from build123d import *

# Parameters (mm, degrees)
SKETCH_1_R          = 1.2
EXTRUDE_1_DEPTH     = 3
EXTRUDE_2_DEPTH     = 200
FILLET_1_R          = 4
SKETCH_4_W          = 24.434656606
SKETCH_4_H          = 24.505426632
CUT_EXTRUDE_1_DEPTH = 4
FILLET_3_R          = 8
SKETCH_5_W          = 15
SKETCH_5_H          = 20
CUT_EXTRUDE_2_DEPTH = 10
FILLET_4_R          = 10
FILLET_5_R          = 10


with BuildPart() as part:
    # 草图1 → 凸台-拉伸1 (new body)
    with BuildSketch(Plane.XY):
        Polygon((-68.534318099, 4.283164377), (-80.94435421, -20.816457208), (-55.844732625, -33.22649332), (-43.434696514, -8.126871734), align=None)
        with Locations((-66.577549394, -0.711768645)):
            Circle(SKETCH_1_R, mode=Mode.SUBTRACT)
        with Locations((-75.441860902, -18.640069777)):
            Circle(SKETCH_1_R, mode=Mode.SUBTRACT)
        with Locations((-57.51355977, -27.504381286)):
            Circle(SKETCH_1_R, mode=Mode.SUBTRACT)
        with Locations((-48.649248262, -9.576080153)):
            Circle(SKETCH_1_R, mode=Mode.SUBTRACT)
    extrude(amount=EXTRUDE_1_DEPTH)

    # 草图2 → 凸台-拉伸2 (add)
    with BuildSketch(Plane.XY.offset(3)):
        Polygon((-86.606649797, -63.783530386), (-38.474241258, 35.126889936), (-35.77668434, 33.814187885), (-83.909092879, -65.096232437), align=None)
    extrude(amount=EXTRUDE_2_DEPTH)

    # 圆角1
    fillet_1_edges = [part.edges().sort_by_distance(p)[0] for p in [
        (-59.839316246, -15.633681193, 3),
        (-62.528614635, -14.304008154, 3),
    ]]
    fillet(fillet_1_edges, radius=FILLET_1_R)

    # 草图4 → 切除-拉伸1 (cut)
    with BuildSketch(Plane(origin=(-44.928588602, 21.863431321, 0), x_dir=(0, 0, 1), z_dir=(-0.8991856392880848, 0.43756735035658034, 0))):
        with Locations((15.217328303, -82.996763505)):
            Rectangle(SKETCH_4_W, SKETCH_4_H)
    extrude(amount=-CUT_EXTRUDE_1_DEPTH, mode=Mode.SUBTRACT)

    # 圆角3
    fillet_3_edges = [part.edges().sort_by_distance(p)[0] for p in [
        (-74.535096738, -42.4049537, 3),
        (-74.535096738, -42.4049537, 27.434656606),
    ]]
    fillet(fillet_3_edges, radius=FILLET_3_R)

    # 草图5 → 切除-拉伸2 (cut)
    with BuildSketch(Plane(origin=(-42.231031684, 20.55072927, 0), x_dir=(0, 0, -1), z_dir=(0.8991856392880848, -0.4375673503565804, 0))):
        with Locations((-60.064574797, -10.249476821)):
            Rectangle(SKETCH_5_W, SKETCH_5_H)
        with Locations((-29.955718497, -10.249476821)):
            Rectangle(SKETCH_5_W, SKETCH_5_H)
        with Locations((-90.173431098, -10.249476821)):
            Rectangle(SKETCH_5_W, SKETCH_5_H)
        with Locations((-120.282287399, -10.249476821)):
            Rectangle(SKETCH_5_W, SKETCH_5_H)
        with Locations((-150.391143699, -10.249476821)):
            Rectangle(SKETCH_5_W, SKETCH_5_H)
        with Locations((-180.5, -10.249476821)):
            Rectangle(SKETCH_5_W, SKETCH_5_H)
        with Locations((-60.064574797, -40.249476821)):
            Rectangle(SKETCH_5_W, SKETCH_5_H)
        with Locations((-90.173431098, -40.249476821)):
            Rectangle(SKETCH_5_W, SKETCH_5_H)
        with Locations((-120.282287399, -40.249476821)):
            Rectangle(SKETCH_5_W, SKETCH_5_H)
        with Locations((-150.391143699, -40.249476821)):
            Rectangle(SKETCH_5_W, SKETCH_5_H)
        with Locations((-180.5, -40.249476821)):
            Rectangle(SKETCH_5_W, SKETCH_5_H)
        with Locations((-60.064574797, -70.249476821)):
            Rectangle(SKETCH_5_W, SKETCH_5_H)
        with Locations((-90.173431098, -70.249476821)):
            Rectangle(SKETCH_5_W, SKETCH_5_H)
        with Locations((-120.282287399, -70.249476821)):
            Rectangle(SKETCH_5_W, SKETCH_5_H)
        with Locations((-150.391143699, -70.249476821)):
            Rectangle(SKETCH_5_W, SKETCH_5_H)
        with Locations((-180.5, -70.249476821)):
            Rectangle(SKETCH_5_W, SKETCH_5_H)
        with Locations((-29.955718497, -40.249476821)):
            Rectangle(SKETCH_5_W, SKETCH_5_H)
    extrude(amount=-CUT_EXTRUDE_2_DEPTH, mode=Mode.SUBTRACT)

    # 圆角4
    fillet_4_edges = [part.edges().sort_by_distance(p)[0] for p in [
        (-37.125462799, 34.470538911, 203),
    ]]
    fillet(fillet_4_edges, radius=FILLET_4_R)

    # 圆角5
    fillet_5_edges = [part.edges().sort_by_distance(p)[0] for p in [
        (-37.125462799, 34.470538911, 3),
    ]]
    fillet(fillet_5_edges, radius=FILLET_5_R)


solid = part.part
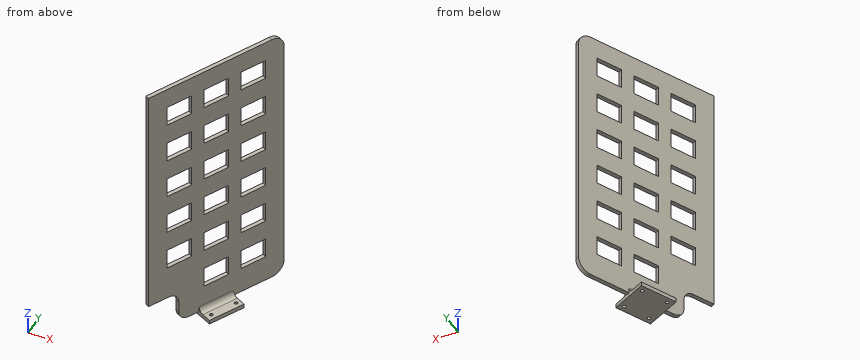
Source: CAD feature listing. Evaluate the final solid. Frame: model axes, mm. Give positions to 0.01 mm unless a question says otherwise; leave off trailing zeros. Write each loop counter-clockwise with the first axis right and the second up, starting at its lowest first coordinate (ties: lowest second). Pieces come first, ordered by that corner, then holes. Notation, with made-up numbers: M -17.75,-18 L -0.75,-18 A18 ccw -0.75,-6 Z; hole C 81.5,39 d4. An arc over 180 degrees is marked long. Return JSON: item names as keys, results as strings. Group by question number.
1) Cut plane B-B, the plane y = 15. Output: boundary loops of the cut face in (x, z), plus the area to 3 significant figures.
2) Pin query (flat end, axial travel): P1, Ø3, axis at x = -48.65, y = -9.58, coming from the +Z side; P2, Ø3.5, axis at x = -45.5, y = 11, coming from the -Z side; P3, Ø3.5, axis at x = -74.5, y = -42.5, coming from the -Z side. Return the tip coordinate at first contact, or that it passes through.
3) Cut plane A-A, the plane z = 151. Output: boundary loops of the cut face in (x, y), plus the area to 3 significant figures.
4) Material intervals for line 1 along Z through (x, y) = (-76, -46); line 2 along Z through (x, y) = (-75, -16); line 3 along X through (y, z) = (-11.5, 137.5), sorted ascending. Write a range as [from, to].
Recorded:
{
 "1": {"outline": "M -48.27,3 L -44.93,3 L -44.93,22.46 L -48.27,22.46 Z; M -48.27,37.46 L -44.93,37.46 L -44.93,52.56 L -48.27,52.56 Z; M -48.27,67.56 L -44.93,67.56 L -44.93,82.67 L -48.27,82.67 Z; M -48.27,97.67 L -44.93,97.67 L -44.93,112.78 L -48.27,112.78 Z; M -48.27,127.78 L -44.93,127.78 L -44.93,142.89 L -48.27,142.89 Z; M -48.27,157.89 L -44.93,157.89 L -44.93,173 L -48.27,173 Z; M -48.27,188 L -44.93,188 L -44.93,203 L -48.27,203 Z", "area": "367 mm²"},
 "2": {"P1": "stops at z = 3", "P2": "stops at z = 3", "P3": "stops at z = 6.1"},
 "3": {"outline": "M -86.61,-63.78 L -83.91,-65.1 L -77.35,-51.61 L -80.04,-50.3 Z; M -71.29,-32.31 L -68.59,-33.62 L -64.22,-24.63 L -66.92,-23.32 Z; M -58.16,-5.34 L -55.47,-6.65 L -51.09,2.34 L -53.79,3.66 Z; M -45.04,21.64 L -42.34,20.33 L -35.78,33.81 L -38.47,35.13 Z", "area": "150 mm²"},
 "4": {"line 1": "z = [26.29, 52.56], [67.56, 82.67], [97.67, 112.78], [127.78, 142.89], [157.89, 173], [188, 203]", "line 2": "z = [0, 3]", "line 3": "x = [-61.16, -57.83]"}
}
